```python
from build123d import *

# Parameters (mm, degrees)
BOSS_EXTRUDE1_DEPTH     = 4
BOSS_EXTRUDE2_START     = -45
BOSS_EXTRUDE2_DEPTH     = 3
BOSS_EXTRUDE3_START     = -39
BOSS_EXTRUDE3_DEPTH     = 3
BOSS_EXTRUDE4_REACH     = 213.107
SKETCH6_R               = 2.5
SKETCH7_W               = 20
SKETCH7_H               = 6
CUT_EXTRUDE1_DEPTH      = 10
CUT_EXTRUDE2_DEPTH      = 228.268563733
FILLET1_R               = 10
CUT_EXTRUDE3_DEPTH      = 228.268563733
SKETCH12_W              = 23
SKETCH12_H              = 10
CUT_EXTRUDE6_DEPTH      = 21
BOSS_EXTRUDE5_REACH     = 213.407
SKETCH13_R              = 2.35
CUT_EXTRUDE7_DEPTH      = 209.214432859
CUT_EXTRUDE7_DEPTH_BACK = 209.214432859
SKETCH15_W              = 6
SKETCH15_H              = 4.56544039
SKETCH15_H_2            = 4.038157292
BOSS_EXTRUDE6_DEPTH     = 1


with BuildPart() as part:
    # Sketch1 → Boss-Extrude1 (new body)
    with BuildSketch(Plane(origin=(0, 0, 0), x_dir=(1, 0, 0), z_dir=(0, 1, 0))):
        with BuildLine():
            Line((-110, 0), (0, 0))
            Line((0, 0), (0, -105))
            Line((0, -105), (-110, -105))
            add(Edge.make_bspline(
                [(-190, -72.5), (-172.262756658, -100.700379519), (-139.265999107, -104.836107107), (-110, -105)],
                knots=[0, 0, 0, 0, 1, 1, 1, 1], degree=3))
            Line((-190, -72.5), (-190, -32.5))
            add(Edge.make_bspline(
                [(-190, -32.5), (-171.707374586, -4.618888995), (-138.989901699, -2.178666842), (-110, 0)],
                knots=[0, 0, 0, 0, 1, 1, 1, 1], degree=3))
        make_face()
    extrude(amount=BOSS_EXTRUDE1_DEPTH)

    # Sketch2 → Boss-Extrude2 (add, symmetric)
    with BuildSketch(Plane.XY.offset(105).offset(BOSS_EXTRUDE2_START)):
        Polygon((-190, 4), (-201, 4), (-201, -11), (-191, -11), (-178, 0), align=None)
    boss_extrude2 = extrude(amount=BOSS_EXTRUDE2_DEPTH, both=True)

    # Mirror1: Boss-Extrude2 across plane
    add(boss_extrude2.mirror(Plane.XY.offset(52.5)))

    # Sketch5 → Boss-Extrude3 (add, symmetric)
    with BuildSketch(Plane.XY.offset(105).offset(BOSS_EXTRUDE3_START)):
        Polygon((-16.979807258, 4), (-7.979807258, 14), (0, 14), (0, 4), align=None)
    boss_extrude3 = extrude(amount=BOSS_EXTRUDE3_DEPTH, both=True)

    # Mirror4: Boss-Extrude3 across plane
    add(boss_extrude3.mirror(Plane.XY.offset(52.5)))

    # Sketch6 → Boss-Extrude4 (add, up to next)
    with BuildSketch(Plane.XY.offset(42), mode=Mode.PRIVATE) as boss_extrude4_sk1:
        with Locations(Location((-4, 10, 0), (0, 0, 180))):
            Circle(SKETCH6_R)
    boss_extrude4_tool1 = extrude(boss_extrude4_sk1.sketch, amount=BOSS_EXTRUDE4_REACH, mode=Mode.PRIVATE) - part.part
    add(boss_extrude4_tool1.solids().sort_by_distance((-4, 10, 42))[0])

    # Sketch7 → Cut-Extrude1 (cut)
    with BuildSketch(Plane(origin=(0, 4, 0), x_dir=(1, 0, 0), z_dir=(0, 1, 0))):
        with Locations((-98, -98.5)):
            Rectangle(SKETCH7_W, SKETCH7_H)
    cut_extrude1 = extrude(amount=-CUT_EXTRUDE1_DEPTH, mode=Mode.SUBTRACT)

    # Mirror5: Cut-Extrude1 across plane
    add(cut_extrude1.mirror(Plane.XY.offset(52.5)), mode=Mode.SUBTRACT)

    # Sketch10 → Cut-Extrude2 (cut, symmetric)
    with BuildSketch(Plane(origin=(0, 4, 0), x_dir=(1, 0, 0), z_dir=(0, 1, 0))):
        Polygon((0, -19), (-39.5, -19), (-48, 0), (0, 0), align=None)
    cut_extrude2 = extrude(amount=CUT_EXTRUDE2_DEPTH, both=True, mode=Mode.SUBTRACT)

    # Mirror6: Cut-Extrude2 across plane
    add(cut_extrude2.mirror(Plane.XY.offset(52.5)), mode=Mode.SUBTRACT)

    # Fillet1
    fillet1_edges = [part.edges().sort_by_distance(p)[0] for p in [
        (-48, 2, 0),
        (-48, 2, 105),
    ]]
    fillet(fillet1_edges, radius=FILLET1_R)

    # Sketch11 → Cut-Extrude3 (cut, symmetric)
    with BuildSketch(Plane(origin=(0, 4, 0), x_dir=(1, 0, 0), z_dir=(0, 1, 0))):
        Polygon((-4.5, -19), (-10.25, -29), (-23.25, -29), (-29, -19), align=None)
    cut_extrude3 = extrude(amount=CUT_EXTRUDE3_DEPTH, both=True, mode=Mode.SUBTRACT)

    # Mirror7: Cut-Extrude3 across plane
    add(cut_extrude3.mirror(Plane.XY.offset(52.5)), mode=Mode.SUBTRACT)

    # Sketch12 → Cut-Extrude6 (cut)
    with BuildSketch(Plane(origin=(0, 0, 0), x_dir=(0, 0, -1), z_dir=(1, 0, 0))):
        with Locations((-52.5, 9)):
            Rectangle(SKETCH12_W, SKETCH12_H)
    extrude(amount=-CUT_EXTRUDE6_DEPTH, mode=Mode.SUBTRACT)

    # Sketch13 → Boss-Extrude5 (add, up to next)
    with BuildSketch(Plane(origin=(0, 0, 64), x_dir=(-1, 0, 0), z_dir=(0, 0, -1)), mode=Mode.PRIVATE) as boss_extrude5_sk1:
        with Locations(Location((3.989903629, 9, 0), (0, 0, 180))):
            Circle(SKETCH13_R)
    boss_extrude5_tool1 = extrude(boss_extrude5_sk1.sketch, amount=BOSS_EXTRUDE5_REACH, mode=Mode.PRIVATE) - part.part
    add(boss_extrude5_tool1.solids().sort_by_distance((-3.989904, 9, 64))[0])

    # Sketch14 → Cut-Extrude7 (cut, two sides: drawn at the far end of the back side and taken through both)
    with BuildSketch(Plane.XY.offset(52.5).offset(-CUT_EXTRUDE7_DEPTH_BACK)):
        with BuildLine():
            Line((-198.09573372, 4), (-198.09573372, -0.56544039))
            ThreePointArc((-198.09573372, -0.56544039), (-191.693337136, -3.763641549), (-198.09573372, -6.961842708))
            Line((-198.09573372, -6.961842708), (-198.09573372, -11))
            Line((-198.09573372, -11), (-202.719197906, -12.115187625))
            Line((-202.719197906, -12.115187625), (-202.588499271, 4.842960165))
            Line((-202.588499271, 4.842960165), (-198.09573372, 4))
        make_face()
    extrude(amount=CUT_EXTRUDE7_DEPTH + CUT_EXTRUDE7_DEPTH_BACK, mode=Mode.SUBTRACT)

    # Sketch15 → Boss-Extrude6 (add)
    with BuildSketch(Plane.ZY.offset(198.09573372)):
        with Locations((60, 1.717279805)):
            Rectangle(SKETCH15_W, SKETCH15_H)
        with Locations((45, 1.717279805)):
            Rectangle(SKETCH15_W, SKETCH15_H)
        with Locations((45, -8.980921354)):
            Rectangle(SKETCH15_W, SKETCH15_H_2)
        with Locations((60, -8.980921354)):
            Rectangle(SKETCH15_W, SKETCH15_H_2)
    extrude(amount=BOSS_EXTRUDE6_DEPTH)


solid = part.part
```
Geometry check sheet. Reference: the model listing, model coordinates, mm. A direction names the side the tool comes from. Coordinates: 2 decimals unless noted, no trailing zeros. Write each loop counter-clockwise with the first axis right and the second up, starting at its lowest first coordinate (ties: lowest second). Pieces come first, ordered by that corner, then holes. Notation, with made-up numbers: M 77.5,16 L 124.5,16 A25 ccw 124.5,33 Z; hole C 43,69 d9. An arc over 180 degrees is marked long. Answer as a JSON object with one key per item and string values.
1. Scan lines: L1, parallel to X at y = 2.75, z = 70; L2, parallel to X at y = -0.5, z = 60; L3, parallel to Y at x = -179.5, z = 50. Record each from-to range of solid material in increasing order.
Answers below:
{"L1": "x = -190 to 0", "L2": "x = -199.1 to -198.01, -193.38 to -178.59", "L3": "y = 0 to 4"}
2. Section check A-A, the plane z = 38. Enter the section's corners in (x, y).
Answers below:
{"outline": "M -190,0 L 0,0 L 0,14 L -7.98,14 L -16.98,4 L -190,4 Z"}
3. Tool access check on faces 4 (the flat face through (-191, -4, 57)), 5 (the flat face through (-17, 2, 29)), 6 (the flat face through (-34, 2, 19)), 7 (the flat face through (-190, 2, 68)), 8 (the flat face through (-190, 2, 37)). Record the directions out of +Z, -Z, +X, -X, +Y, -Y that give a thin tool (end or side, any length) a straight path to the whole face; none if there is none.
Answers below:
{"face 4": "-X, -Y", "face 5": "-Z, +Y, -Y", "face 6": "-Z, +X, +Y, -Y", "face 7": "+Z, -X, +Y, -Y", "face 8": "-Z, -X, +Y, -Y"}
4. Draft check along X on faces 1 (the flat face through (-98, 2, 95.5)), 2 (the cylindrical face through (-2.906, 11.085, 52.661)), 3 (the flat face through (-6, 9, 69)). Enter one of: released by +X, released by -X, zero draft, split by the parting line, or undercut.
Answers below:
{"face 1": "undercut", "face 2": "split by the parting line", "face 3": "zero draft"}
5. Section check B-B, the plane y = 9. Enter the section's corners in (x, z), plus the area to 3 significant figures.
Answers below:
{"outline": "M -12.48,36 L 0,36 L 0,41 L -1.64,41 L -1.64,64 L 0,64 L 0,69 L -12.48,69 L -12.48,64 L -6.34,64 L -6.34,41 L -12.48,41 Z", "area": "233 mm²"}
6. Go/stop test with flat-tipped pins: pin 1 Ø4.5 at (x, y) = (-193, -4) entering from -Z; pin 2 Ø3 at (x, z) = (-96.5, 16) entering from +Y; pin 3 Ø6 at (x, z) = (-96.5, 23) entering from -Y. Record where each tip stops, or that it passes through.
Answers below:
{"pin 1": "stops at z = 42", "pin 2": "stops at y = 4", "pin 3": "stops at y = 0"}
